The listing builds one solid part. Answer for the finished solid, in the listing's coordinates (mm). Face numbers are marked on the shaded views. A direction names the side the tool comes from. Round coordinates to 2 decimals unless told otherwise and drop trailing zeros. Write each loop counter-clockwise with the first axis right and the second up, starting at its lowest first coordinate (ties: lowest second). Pieces come first, ordered by that corner, then holes. Notation, with made-up numbers: (70.25, 30.5) - (105.25, 30.5) arc R12 ccw to (105.25, 35.5) - close; hole circle Ø2 at (19.5, 45.5). An arc over 180 degrees is marked (long way). Return JSON: item names as keys, results as strings. Group by question number.
Autodesk Inventor part; units mm, degrees
ref_plane "YZ Plane" through (0, 0, 0) normal (1, 0, 0) x (0, 1, 0)
ref_plane "XZ Plane" through (0, 0, 0) normal (0, 1, 0) x (-1, 0, 0)
ref_plane "XY Plane" through (0, 0, 0) normal (0, 0, 1) x (1, 0, 0)
sketch "Sketch4" plane through (0, 0, 0) normal (0, 1, 0) x (-1, 0, 0)
  line L0 (0, 0) -> (100, 0)
  line L1 (100, 0) -> (100, -220)
  line L2 (100, -220) -> (0, -220)
  line L3 (0, -220) -> (0, 0)
  dimension "d12" = 100
  dimension "d13" = 220
extrude "Extrusion4" add sketch "Sketch4" along normal blind 5
sketch "Sketch5" plane through (0, 5, 0) normal (0, 1, 0) x (1, 0, 0)
  line L0 (-100, 220) -> (-100, 0)
  line L1 (-100, 0) -> (0, 0)
  line L2 (0, 0) -> (0, 3)
  line L3 (0, 3) -> (-100, 3)
  line L4 (-100, 3) -> (-100, 0)
  line L5 (-100, 220) -> (0, 220)
  line L6 (0, 220) -> (0, 217)
  line L7 (0, 217) -> (-100, 217)
  line L8 (-100, 217) -> (-100, 220)
  point P0 (0, 0)
  point P1 (-100, 217)
  dimension "d16" = 100
  dimension "d17" = 3
  dimension "d18" = 100
  dimension "d19" = 3
extrude "Extrusion5" add sketch "Sketch5" along normal blind 40
properties part number "1P10 DP3 pi holder"
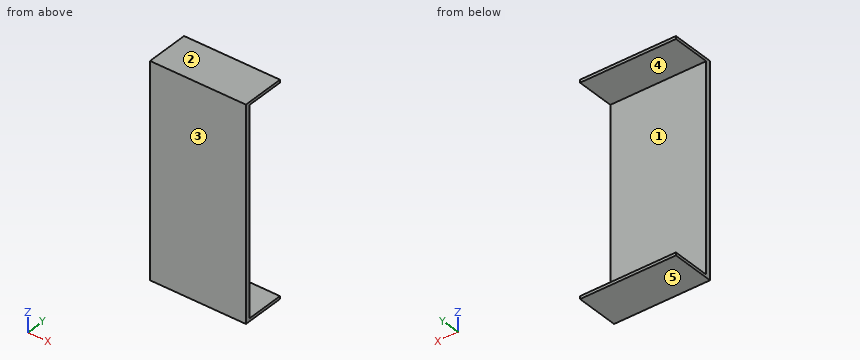
(1) Find section A-A (y = 34.5). Write down the section's boundary in (x, z), plus the area to 3 significant figures.
(2) Consider line 1 (Z direction, x = -90, y = 35.5); line 2 (Y direction, x = -68, z = -48.5). Determine where each line is inside the solid, lowest interval first.
(3) Determine the mould class of the marked faces 3, 4 and 5 for opening direction Z: +Z half, -Z half, draft (parallel to the pull), parting line (faces both ways), or undercut.
(4) Find section C-C (z = -168). Write down the section's boundary in (x, y), plus the area to 3 significant figures.
(5) A flat-ended cylindrical pin translates along its axis: pin 1 (10 mm diameter, centred on x = -75, z = -162.5, fed in from +Y). Find the tip coordinate at first contact, or state that the pin passes through.
(6) For the marked faces 1 and 2, determine the directions among +Z, -Z, +X, -X, +Y, -Y from which every point of the face is accessible in a straight line to the end or side of a thin tool.
(7) Find section B-B (x = -83). Write down the section's boundary in (y, z).
Check sheet entries:
{
 "1": {"outline": "(-100, -220) - (0, -220) - (0, -217) - (-100, -217) - close; (-100, -3) - (0, -3) - (0, 0) - (-100, 0) - close", "area": "600 mm^2"},
 "2": {"line 1": "z = -220 to -217, -3 to 0", "line 2": "y = 0 to 5"},
 "3": {"face 3": "draft", "face 4": "undercut", "face 5": "-Z half"},
 "4": {"outline": "(-100, 0) - (0, 0) - (0, 5) - (-100, 5) - close", "area": "500 mm^2"},
 "5": {"pin 1": "stops at y = 5"},
 "6": {"face 1": "+X, -X, +Y", "face 2": "+Z, +X, -X, +Y, -Y"},
 "7": {"outline": "(0, -220) - (45, -220) - (45, -217) - (5, -217) - (5, -3) - (45, -3) - (45, 0) - (0, 0) - close"}
}
